```python
from build123d import *

# Parameters (mm, degrees)
SKETCH1_W           = 76.2
SKETCH1_H           = 46.228
SKETCH1_R           = 1.6
SKETCH1_R_2         = 11.049
BOSS_EXTRUDE1_DEPTH = 4.7625
FILLET1_R           = 3.81


with BuildPart() as part:
    # Sketch1 → Boss-Extrude1 (new body)
    with BuildSketch(Plane(origin=(0, 0, 0), x_dir=(1, 0, 0), z_dir=(0, 1, 0))):
        with Locations((38.1, 23.114)):
            Rectangle(SKETCH1_W, SKETCH1_H)
        with Locations(Location((68.58, 38.608, 0), (0, 0, 90))):
            Circle(SKETCH1_R, mode=Mode.SUBTRACT)
        with Locations(Location((7.62, 38.608, 0), (0, 0, 90))):
            Circle(SKETCH1_R, mode=Mode.SUBTRACT)
        with Locations(Location((68.58, 7.62, 0), (0, 0, 90))):
            Circle(SKETCH1_R, mode=Mode.SUBTRACT)
        with Locations(Location((7.62, 7.62, 0), (0, 0, 90))):
            Circle(SKETCH1_R, mode=Mode.SUBTRACT)
        with Locations(Location((38.1, 23.114, 0), (0, 0, 90))):
            Circle(SKETCH1_R_2, mode=Mode.SUBTRACT)
        with Locations(Location((22.606, 38.608, 0), (0, 0, 90))):
            Circle(SKETCH1_R, mode=Mode.SUBTRACT)
        with Locations(Location((53.594, 38.608, 0), (0, 0, 90))):
            Circle(SKETCH1_R, mode=Mode.SUBTRACT)
        with Locations(Location((22.606, 7.62, 0), (0, 0, 90))):
            Circle(SKETCH1_R, mode=Mode.SUBTRACT)
        with Locations(Location((53.594, 7.62, 0), (0, 0, 90))):
            Circle(SKETCH1_R, mode=Mode.SUBTRACT)
    extrude(amount=BOSS_EXTRUDE1_DEPTH)

    # Fillet1
    fillet1_edges = [part.edges().sort_by_distance(p)[0] for p in [
        (0, 2.38125, -46.228),
        (76.2, 2.38125, -46.228),
        (76.2, 2.38125, 0),
        (0, 2.38125, 0),
    ]]
    fillet(fillet1_edges, radius=FILLET1_R)


solid = part.part
```
For this review, take the finished solid that the model builds, in its own axes (mm). Round coordinates to 2 decimals unless told otherwise and drop trailing zeros. Write each loop counter-clockwise with the first axis right and the second up, starting at its lowest first coordinate (ties: lowest second). Pieces come first, ordered by that corner, then holes. Notation, with made-up numbers: (-37, 10.5) -> (5, 10.5) arc R32 ccw to (5, 36.5) -> close; hole circle Ø4 at (89.5, 79.5). An arc over 180 degrees is marked (long way). One line per question, with ' | ' between items. Start each with the question number.
(1) Add section B-B, the plane x = 38.1. Write out the cut boundary in (y, z) (1 decimal), plus the area to 3 significant figures.
(2) Add section D-D, the plane y = 3.3. Give the number of separate pieces and of enclosed holes in the cut face, plus the area to 3 significant figures.
(3) Add section C-C, the plane x = 68.58. Write out the cut boundary in (y, z).
(4) Add section A-A, the plane z = -7.62. Write out the cut boundary in (x, y).
(5) For line 1 along Z through (x, y) = (7.62, 2.9); line 2 along X through (y, z) = (3.25, -7.62); line 3 along X through (y, z) = (4.3, -8), list the stretches that pass through material, from the lowest coordinate up. Write a range as from..to.
(6) Mouldability with a two-part tool opening along Z and no side actions: class faces 1 (the face through (67.23, 2.35, -8.48)), 2 (the face through (67.23, 2.35, -39.47)), 3 (the face through (38, 2, 0)), 4 (the face through (38, 2, -46.228)) as released by +Z, released by -Z, zero draft, split by the parting line, or undercut.
Answer list:
1) outline: (0, -46.2) -> (4.8, -46.2) -> (4.8, -34.2) -> (0, -34.2) -> close; (0, -12.1) -> (4.8, -12.1) -> (4.8, 0) -> (0, 0) -> close | area: 115 mm²
2) separate pieces: 1 | enclosed holes: 9 | area: 3,060 mm²
3) outline: (0, -46.23) -> (4.76, -46.23) -> (4.76, -40.21) -> (0, -40.21) -> close; (0, -37.01) -> (4.76, -37.01) -> (4.76, -9.22) -> (0, -9.22) -> close; (0, -6.02) -> (4.76, -6.02) -> (4.76, 0) -> (0, 0) -> close
4) outline: (0, 0) -> (6.02, 0) -> (6.02, 4.76) -> (0, 4.76) -> close; (9.22, 0) -> (21.01, 0) -> (21.01, 4.76) -> (9.22, 4.76) -> close; (24.21, 0) -> (51.99, 0) -> (51.99, 4.76) -> (24.21, 4.76) -> close; (55.19, 0) -> (66.98, 0) -> (66.98, 4.76) -> (55.19, 4.76) -> close; (70.18, 0) -> (76.2, 0) -> (76.2, 4.76) -> (70.18, 4.76) -> close
5) line 1: -46.23..-40.21, -37.01..-9.22, -6.02..0 | line 2: 0..6.02, 9.22..21.01, 24.21..51.99, 55.19..66.98, 70.18..76.2 | line 3: 0..6.07, 9.17..21.05, 24.16..52.04, 55.15..67.03, 70.13..76.2
6) face 1: undercut | face 2: undercut | face 3: released by +Z | face 4: released by -Z
